from build123d import *

# Parameters (mm, degrees)
SKETCH1_R           = 59.69
DOME_BASE_DEPTH     = 9.525
DOME1_FACE_RADIUS   = 59.69
DOME1_HEIGHT        = 30.48
SKETCH2_R           = 64.77
SKETCH2_R_2         = 59.69
BOSS_EXTRUDE2_DEPTH = 1.905
SKETCH3_R           = 2.921
CUT_EXTRUDE1_DEPTH  = 100.206430235


# Read off the part's stored shape, not the designer's step: Shell1
with BuildPart() as part:
    # Sketch1 → Dome Base (new body)
    with BuildSketch(Plane(origin=(0, 0, 0), x_dir=(1, 0, 0), z_dir=(0, 1, 0))):
        with Locations(Location((0, 0, 0), (0, 0, 90))):
            Circle(SKETCH1_R)
    extrude(amount=DOME_BASE_DEPTH)

    # Dome1: a dome of height H over a round flat face of radius A is a cap of a sphere of radius (A * A + H * H) / (2 * H)
    dome1_r = (DOME1_FACE_RADIUS * DOME1_FACE_RADIUS + DOME1_HEIGHT * DOME1_HEIGHT) / (2 * DOME1_HEIGHT)
    dome1_base = Plane((0, 9.525, 0), z_dir=(0, 1, 0))
    with Locations(dome1_base.offset(DOME1_HEIGHT - dome1_r)):
        dome1_ball = Sphere(dome1_r, mode=Mode.PRIVATE)
    add(split(dome1_ball, bisect_by=dome1_base, keep=Keep.TOP, mode=Mode.PRIVATE))

    # Shell1 outline → Shell1 (revolve, cut)
    with BuildSketch(Plane.XY):
        with BuildLine():
            Line((57.785, 0), (57.785000043, 8.9034161))
            ThreePointArc((57.785000043, 8.9034161), (32.371077914, 30.386404711), (0, 38.1))
            Line((0, 38.1), (0, 0))
            Line((0, 0), (57.785, 0))
        make_face()
    revolve(axis=Axis((0, 0, 0), (0, 1, 0)), mode=Mode.SUBTRACT)

    # Sketch2 → Boss-Extrude2 (add)
    with BuildSketch(Plane.XZ):
        with Locations(Location((0, 0, 0), (0, 0, 270))):
            Circle(SKETCH2_R)
        with Locations(Location((0, 0, 0), (0, 0, 270))):
            Circle(SKETCH2_R_2, mode=Mode.SUBTRACT)
    extrude(amount=-BOSS_EXTRUDE2_DEPTH)

    # Sketch3 → Cut-Extrude1 (cut, through all)
    with BuildSketch(Plane(origin=(0, 1.905, 0), x_dir=(1, 0, 0), z_dir=(0, 1, 0))):
        with Locations((-53.788136875, -34.930424511)):
            Circle(SKETCH3_R)
        with Locations((51.220488437, -38.59740651)):
            Circle(SKETCH3_R)
        with Locations((-41.225183347, 49.130260359)):
            Circle(SKETCH3_R)
        with Locations((43.739964823, 46.905369653)):
            Circle(SKETCH3_R)
    extrude(amount=-CUT_EXTRUDE1_DEPTH, mode=Mode.SUBTRACT)


solid = part.part
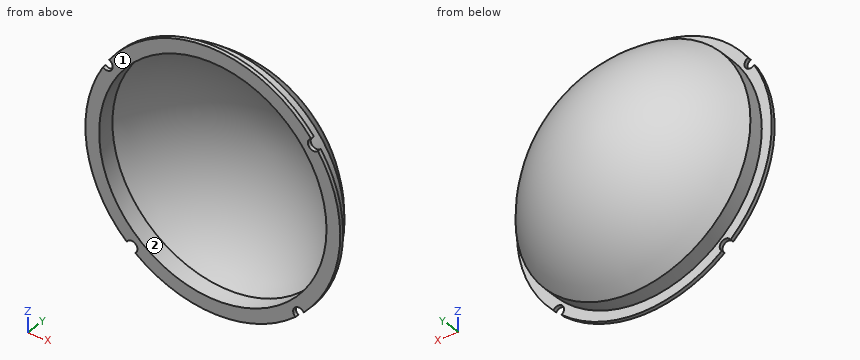
Geometry check sheet. Reference: the model listing, model coordinates, mm. Face numbers are marked on the shaded views. Give positions to 0.01 mm unless a question says otherwise; leave off trailing zeros. Order: outer loops, then holes, each group sorted by start corner. A loop starts at its lowest first (then second) coordinate and runs counter-clockwise, first axis right, second up. Notation, with made-up numbers: M 10,12.25 L 64,12.25 A23 cw 64,49.25 Z; hole C 64.25,33 d6. An arc over 180 degrees is marked long. Use a Markdown table: item, result.
Item 1: Material ranges on line 1 along X through (y, z) = (2, 0) (3 decimals); line 2 along X through (y, z) = (19.5, 33), recorded low to high.
Answers follow:
| item | result |
|---|---|
| line 1 | x = -59.69 to -57.785, 57.785 to 59.69 |
| line 2 | x = -38.89 to -35.15, 35.15 to 38.89 |
Item 2: Section check A-A (z = 0). Record the cut outline in (x, y) (3 decimals), and give its area (3 significant figures).
Answers follow:
| item | result |
|---|---|
| outline | M -64.77,0 L -57.785,0 L -57.785,8.903 A71.781 cw 57.785,8.903 L 57.785,0 L 64.77,0 L 64.77,1.905 L 59.69,1.905 L 59.69,9.525 A73.686 ccw -59.69,9.525 L -59.69,1.905 L -64.77,1.905 Z |
| area | 315 mm2 |
Item 3: Section check B-B (x = 0). Record the cut outline in (y, z) (3 decimals), and give its area (3 significant figures).
Answers follow:
| item | result |
|---|---|
| outline | M 0,-64.77 L 1.905,-64.77 L 1.905,-59.69 L 9.525,-59.69 A73.686 ccw 9.525,59.69 L 1.905,59.69 L 1.905,64.77 L 0,64.77 L 0,57.785 L 8.903,57.785 A71.781 cw 8.903,-57.785 L 0,-57.785 Z |
| area | 315 mm2 |
Item 4: Depth check by flat-ended pin: P1, Ø1, axis at x = 27.5, y = 22.5, coming from the +Z side; P2, Ø1.5, axis at x = -36, z = -25, coming from the -Y side; P3, Ø9.5, axis at x = -53.79, z = 34.93, coming from the +Y side; P4, Ø5.5, axis at x = -41.23, z = -49.13, coming from the +Y side. Enter the tip coordinate at first touch or a pass-through.
Answers follow:
| item | result |
|---|---|
| P1 | stops at z = 39.74 |
| P2 | stops at y = 22.58 |
| P3 | stops at y = 9.94 |
| P4 | passes through |
Item 5: Section check C-C (y = 3.5). Record the cut outline in (x, z) (3 decimals), and give its area (3 significant figures).
Answers follow:
| item | result |
|---|---|
| outline | C 0,0 d119.38; hole C 0,0 d115.57 |
| area | 703 mm2 |
Item 6: Draft check along Z on the marked faces 1 and 2. Enter one of: +Z half, -Z half, draft (parallel to the pull), parting line (faces both ways), or undercut.
Answers follow:
| item | result |
|---|---|
| face 1 | draft |
| face 2 | undercut |
